Study the drawing (mm; zero at the part's minimum x, y, z) and answer. A direction names the side the tool comes from. Give positions to 0.01 mm unless a question says otherwise; leave off trailing zeros. Loops run counter-clockwise (first coordinate to the right, second up) from the corner with the lowest first, then second, coordinate; pieces in that order, holes last. Notation, with made-up numbers: M 28.5,-23 L 44.5,-23 A20 cw 44.5,14 Z; hole C 55,28 d8. An arc over 180 degrees is marked long. Return JSON: item names as keys, results as strings.
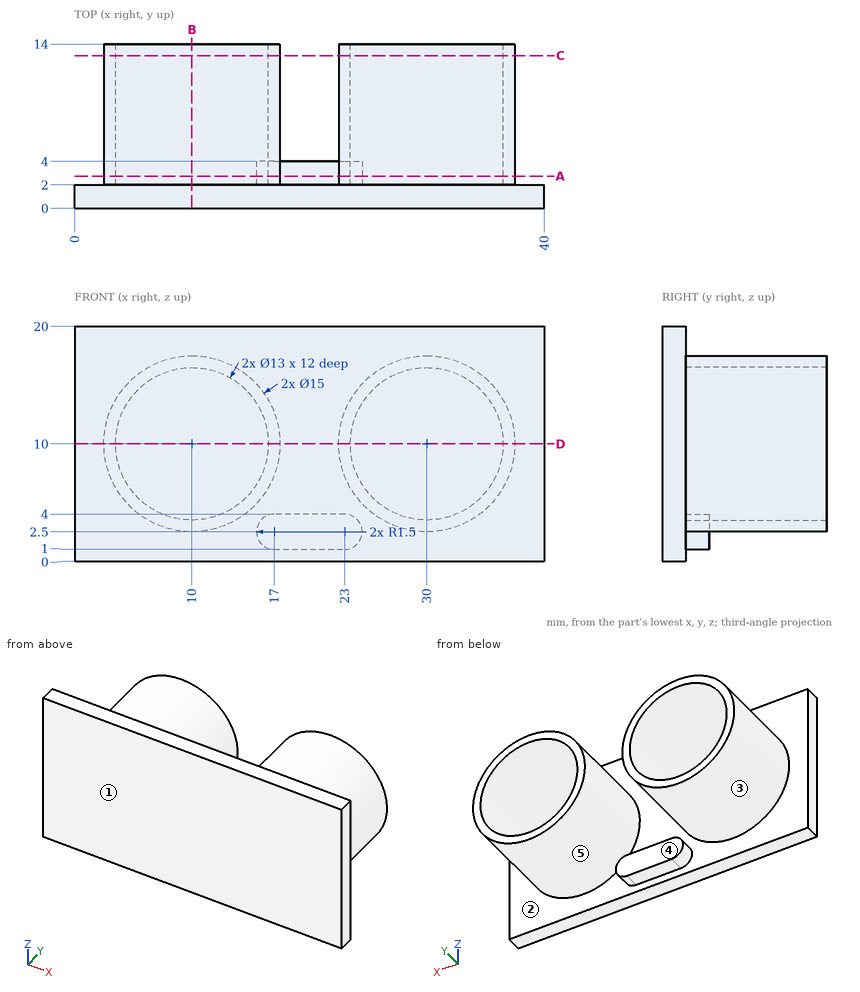
(1) The part is cut by section B-B (x = 10). Determine the outline of the cut face in (y, z), and give its area (3 significant figures).
Values follow:
{"outline": "M 0,0 L 2,0 L 2,2.5 L 14,2.5 L 14,3.5 L 2,3.5 L 2,16.5 L 14,16.5 L 14,17.5 L 2,17.5 L 2,20 L 0,20 Z", "area": "64.0 mm²"}
(2) Straight lines are drawn through the part: line 1 along X through (y, z) = (6.5, 10); line 2 along X through (y, z) = (2.25, 9); line 3 along Y through (x, z) = (21, 12.5). For each, find the intervals that lie inside material, in ascending order.
Values follow:
{"line 1": "2.5 to 3.5, 16.5 to 17.5, 22.5 to 23.5, 36.5 to 37.5", "line 2": "2.57 to 3.58, 16.42 to 17.43, 22.57 to 23.58, 36.42 to 37.43", "line 3": "0 to 2"}
(3) Given pin 1 (4 mm diameter, centred on x = 28, z = 9.5, fed in from +Y); pin 2 (1 mm diameter, centred on x = 10, y = 5.5, fed in from -Z); pin 3 (4 mm diameter, centred on y = 12.5, z = 17, fed in from -X), each flat-ended and moving along its own axis, determine where each tip first touches the part or whether it passes through.
Values follow:
{"pin 1": "y = 2", "pin 2": "z = 2.5", "pin 3": "x = 4.41"}
(4) The part is cut by section D-D (z = 10). Determine the outline of the cut face in (x, y).
Values follow:
{"outline": "M 0,0 L 40,0 L 40,2 L 37.5,2 L 37.5,14 L 36.5,14 L 36.5,2 L 23.5,2 L 23.5,14 L 22.5,14 L 22.5,2 L 17.5,2 L 17.5,14 L 16.5,14 L 16.5,2 L 3.5,2 L 3.5,14 L 2.5,14 L 2.5,2 L 0,2 Z"}
(5) A tool of negligible diameter and unlimited length cuts with its end or side. For the marked faces 4 and 5, from which of +Z, -Z, +X, -X, +Y, -Y can it reach the whole face along a straight path? Write none if from no direction.
Values follow:
{"face 4": "-Z, +Y", "face 5": "+Y"}
(6) The part is cut by section A-A (y = 2.75). Determine the outline of the cut face in (x, z), and give its area (3 significant figures).
Values follow:
{"outline": "C 10,10 d15; M 17,1 L 23,1 A1.5 ccw 23,4 L 17,4 A1.5 ccw Z; C 30,10 d15; hole C 10,10 d13; hole C 30,10 d13", "area": "113 mm²"}
(7) The part is cut by section C-C (y = 13). Determine the outline of the cut face in (x, z), and give its area (3 significant figures).
Values follow:
{"outline": "C 10,10 d15; C 30,10 d15; hole C 10,10 d13; hole C 30,10 d13", "area": "88.0 mm²"}
(8) Determine the mould class of the marked faces 1, 2 and 3 for opening direction X: released by +X, released by -X, zero draft, split by the parting line, or undercut.
Values follow:
{"face 1": "zero draft", "face 2": "undercut", "face 3": "undercut"}
